Geometry: see drawing. Coordinates: mm, zero at the bounding-box minimum. Round coordinates to 2 decimals unless told otherwise and drop trailing zeros. Loops run counter-clockwise (first coordinate to the right, second up) from the corner with the lowest first, then second, coordinate; pieces in that order, holes last.
(1) Cut plane A-A, the plane x = 37.5. Output: boundary loops of the cut face in (y, z), and give its area (3 significant figures).
(2) Cut plane D-D, the plane z = 24. Output: boundary loops of the cut face in (x, y), and give its area (3 significant figures).
(3) Line query: line 1 (Y direction, x = 3, z = 21.5); line 2 (Z direction, x = 4, y = 16); line 3 (X direction, y = 19.5, z = 49.5). Output: solid intervals per line, ascending.
(4) Cut plane B-B, the plane z = 48.5. Output: boundary loops of the cut face in (x, y).
(5) Cut plane C-C, the plane y = 63.5. Output: boundary loops of the cut face in (x, z), and give its area (3 significant figures).
(6) First-contact query: pin 1 Ø3 at (x, z) = (36.5, 39) entering from +Y; pin 2 Ø8 at (x, y) = (31.5, 41.5) entering from +Z. Flat tips, straight axial feed; report the tip coordinate or a pass-through.
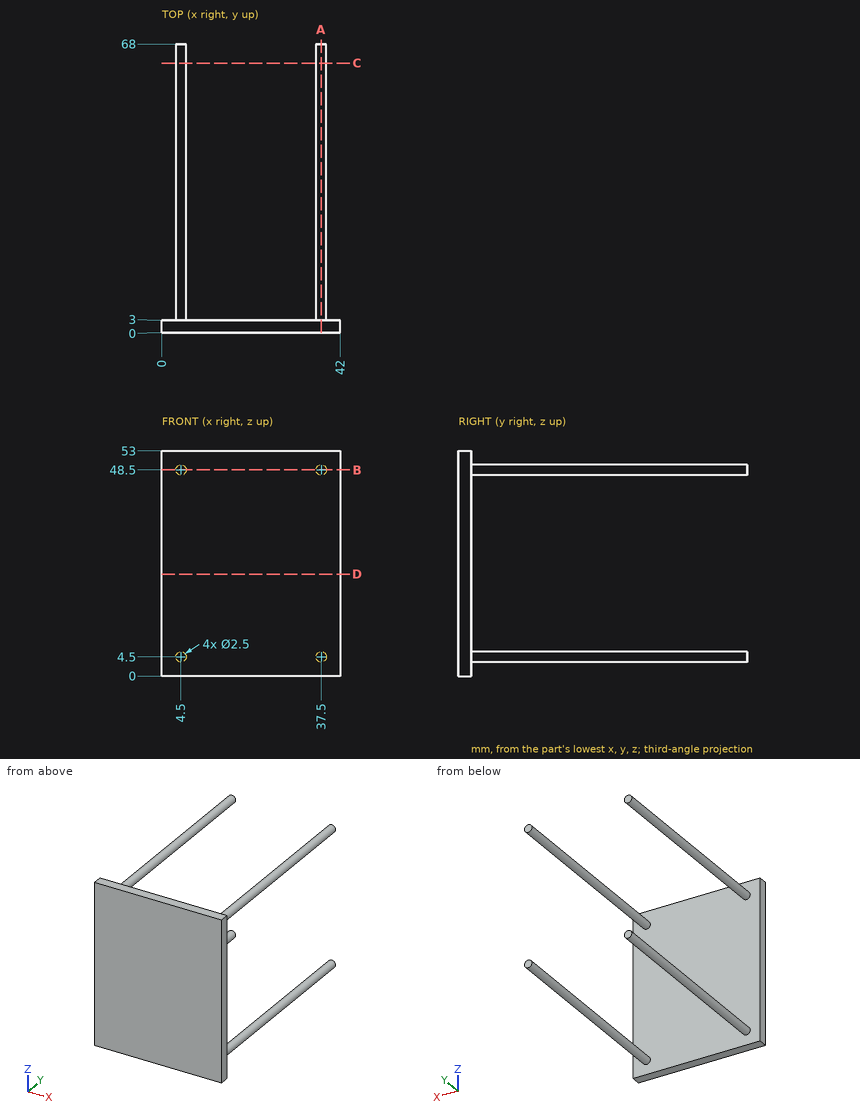
Reported:
1. outline: (0, 0) - (3, 0) - (3, 3.25) - (68, 3.25) - (68, 5.75) - (3, 5.75) - (3, 47.25) - (68, 47.25) - (68, 49.75) - (3, 49.75) - (3, 53) - (0, 53) - close
1. area: 484 mm2
2. outline: (0, 0) - (42, 0) - (42, 3) - (0, 3) - close
2. area: 126 mm2
3. line 1: y = 0 to 3
3. line 2: z = 3.35 to 5.65, 47.35 to 49.65
3. line 3: x = 3.75 to 5.25, 36.75 to 38.25
4. outline: (0, 0) - (42, 0) - (42, 3) - (38.75, 3) - (38.75, 68) - (36.25, 68) - (36.25, 3) - (5.75, 3) - (5.75, 68) - (3.25, 68) - (3.25, 3) - (0, 3) - close
5. outline: circle Ø2.5 at (4.5, 4.5); circle Ø2.5 at (4.5, 48.5); circle Ø2.5 at (37.5, 4.5); circle Ø2.5 at (37.5, 48.5)
5. area: 19.6 mm2
6. pin 1: stops at y = 3
6. pin 2: passes through
